```python
from build123d import *

# Parameters (mm, degrees)
EXTRUDE_1_DEPTH     = 40
FILLET_1_R          = 20
SKETCH_3_R          = 5
CUT_EXTRUDE_1_DEPTH = 10
SKETCH_15_R         = 1.5
CUT_EXTRUDE_2_DEPTH = 10
SKETCH_18_R         = 1.5
CUT_EXTRUDE_5_DEPTH = 10


with BuildPart() as part:
    # 草图1 → 凸台-拉伸1 (new body)
    with BuildSketch(Plane(origin=(0, 0, 0), x_dir=(1, 0, 0), z_dir=(0, 1, 0))):
        Polygon((-2.488479263, -6.032258065), (-32.488479263, -6.032258065), (-32.488479263, 43.967741935), (-30.488479263, 43.967741935), (-30.488479263, -4.032258065), (-2.488479263, -4.032258065), align=None)
    extrude(amount=EXTRUDE_1_DEPTH)

    # 圆角1
    fillet_1_edges = [part.edges().sort_by_distance(p)[0] for p in [
        (-31.488479263, 40, -43.967741935),
        (-31.488479263, 0, -43.967741935),
    ]]
    fillet(fillet_1_edges, radius=FILLET_1_R - 0.0001)  # a hair under: the kernel refuses the full size

    # 草图3 → 切除-拉伸1 (cut)
    with BuildSketch(Plane.ZY.offset(32.488479263)):
        with Locations((-23.967741935, 20)):
            Circle(SKETCH_3_R)
    extrude(amount=-CUT_EXTRUDE_1_DEPTH, mode=Mode.SUBTRACT)

    # 草图15 → 切除-拉伸2 (cut)
    with BuildSketch(Plane(origin=(-32.488479263, 20.448882386, -1043.967741935), x_dir=(0, 0, 1), z_dir=(-1, 0, 0))):
        with Locations((1012, -0.448882386)):
            Circle(SKETCH_15_R)
        with Locations((1020, 7.551117614)):
            Circle(SKETCH_15_R)
        with Locations((1028, -0.448882386)):
            Circle(SKETCH_15_R)
        with Locations((1020, -8.448882386)):
            Circle(SKETCH_15_R)
    extrude(amount=-CUT_EXTRUDE_2_DEPTH, mode=Mode.SUBTRACT)

    # 草图18 → 切除-拉伸5 (cut)
    with BuildSketch(Plane(origin=(0, 0, 4.032258065), x_dir=(-1, 0, 0), z_dir=(0, 0, -1))):
        with Locations((8.988479263, 35)):
            Circle(SKETCH_18_R)
        with Locations((23.988479263, 35)):
            Circle(SKETCH_18_R)
        with Locations((23.988479263, 5)):
            Circle(SKETCH_18_R)
        with Locations((8.988479263, 5)):
            Circle(SKETCH_18_R)
    extrude(amount=-CUT_EXTRUDE_5_DEPTH, mode=Mode.SUBTRACT)


solid = part.part
```
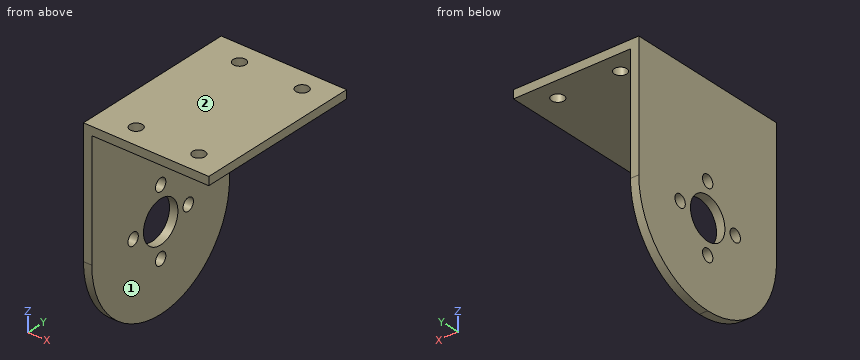
For this review, take the finished solid that the model builds, in its own axes (mm). Face numbers are marked on the shaded views. A direction names the side the tool comes from. Give positions to 0.01 mm unless a question says otherwise; leave off trailing zeros. Write each loop counter-clockwise with the first axis right and the second up, starting at its lowest first coordinate (ties: lowest second). Pieces come first, ordered by that corner, then holes.
Item 1: Take a section at C-C (y = 28). Give the boundary of the cut face in (x, z).
Item 2: Take a section at A-A (y = 5). Give the boundary of the cut face in (x, z), and give its area (3 significant figures).
Item 3: Machinability: for the marked faces 1 and 2, which of the approach directions +Z, -Z, +X, -X, +Y, -Y give a long, thin tool a straight path to every point of the face, cutting with its end or side? Answer none if there is none.
Item 4: Insertion check: P1, Ø2.5, axis at y = 20, z = -15.97, coming from the -X side; P2, Ø5, axis at y = 28.5, z = -38.5, coming from the +X side; P3, Ø10, axis at x = -10.5, y = 23, coming from the -Z side. Each pin has a flat end and moves straight along its axis. Give the tip position at first contact, or say it passes through.
Item 5: Take a section at D-D (x = -29.5). Give the boundary of the cut face in (y, z), and give its area (3 significant figures).
Item 6: Take a section at B-B (z = -28). Give the boundary of the cut face in (x, y).
Item 7: Wall thickness on probe 1 along X at (y, z) = (32, -11); probe 2 along Z at (x, y) = (-5, 32): over which ranges is each line inside the solid? List them lowest first.
Established:
1. outline: (-32.49, -42.3) - (-30.49, -42.3) - (-30.49, -25.47) - (-32.49, -25.47) - close; (-32.49, -22.47) - (-30.49, -22.47) - (-30.49, 4.03) - (-2.49, 4.03) - (-2.49, 6.03) - (-32.49, 6.03) - close
2. outline: (-32.49, -37.2) - (-30.49, -37.2) - (-30.49, 4.03) - (-25.49, 4.03) - (-25.49, 6.03) - (-32.49, 6.03) - close; (-22.49, 4.03) - (-10.49, 4.03) - (-10.49, 6.03) - (-22.49, 6.03) - close; (-7.49, 4.03) - (-2.49, 4.03) - (-2.49, 6.03) - (-7.49, 6.03) - close
2. area: 130 mm2
3. face 1: -Z, +X, +Y, -Y
3. face 2: +Z, +X, -X, +Y, -Y
4. P1: passes through
4. P2: stops at x = -30.49
4. P3: stops at z = 4.03
5. outline: (0, 4.03) - (40, 4.03) - (40, 6.03) - (0, 6.03) - close
5. area: 80.0 mm2
6. outline: (-32.49, 0.41) - (-30.49, 0.41) - (-30.49, 17.04) - (-32.49, 17.04) - close; (-32.49, 22.96) - (-30.49, 22.96) - (-30.49, 39.59) - (-32.49, 39.59) - close
7. probe 1: x = -32.49 to -30.49
7. probe 2: z = 4.03 to 6.03
